Verification items for the finished model (mm, model axes). A direction names the side the tool comes from. Round coordinates to 2 decimals unless told otherwise and drop trailing zeros. Order: outer loops, then holes, each group sorted by start corner. A loop starts at its lowest first (then second) coordinate and runs counter-clockwise, first axis right, second up. Notation, with made-up numbers: M -20.75,-7.75 L 25.25,-7.75 A16 ccw 25.25,13.25 Z; hole C 50.25,8.5 d11. An arc over 180 degrees is marked long. Use one line per item in the form item = value. Start each with the question number.
Item 1: Tool access check on faces 1 (the flat face through (200, -12, -151)), 2 (the flat face through (0, -12, -152)). Record the directions out of +Z, -Z, +X, -X, +Y, -Y that give a thin tool (end or side, any length) a straight path to the whole face; none if there is none.
Item 2: Cross-section at C-C on z = -156. Enter the section's corners in (x, y), then the cut area to 4 significant figures.
Item 3: Thickness scan on probe 1 along X at (y, z) = (-23, -133.5); probe 2 along Z at (x, y) = (142.5, -8.25); probe 3 along Z at (x, y) = (99.5, -19.25). Record the ranges inside material, lowest first. Write a range as [from, to].
Item 4: Release check for a two-part mould opening along Z. For faces 3 (the flat face through (148, -12, -300)), 4 (the flat face through (99, -12, -151)), 5 (the flat face through (81, 0, -148)), 6 (the flat face through (149, -12, -100)) record: +Z half, -Z half, draft (parallel to the pull), parting line (faces both ways), or undercut.
Item 5: Cross-section at A-A on x = 161.5. Enter the section's corners in (y, z), then the cut area to 4 significant figures.
Item 6: Cross-section at B-B on y = -15.5. Enter the section's corners in (x, z).
from build123d import *

# Parameters (mm, degrees)
F0_W     = 300
F0_H     = 300
F0_W_2   = 101
F0_H_2   = 101
F1_DEPTH = 25
F2_SIZE  = 5


with BuildPart() as f1:
    # F0 (on Front) → F1 (new body)
    with BuildSketch(Plane.XZ):
        with Locations((150, -150)):
            Rectangle(F0_W, F0_H)
        with Locations((149.5, -150.5)):
            Rectangle(F0_W_2, F0_H_2, mode=Mode.SUBTRACT)
    extrude(amount=F1_DEPTH)

    # F2
    f2_edges = [f1.edges().sort_by_distance(p)[0] for p in [
        (0, -12.5, -300),
        (300, -12.5, -300),
        (300, -12.5, 0),
        (0, -12.5, 0),
        (200, -12.5, -201),
        (200, -12.5, -100),
        (99, -12.5, -100),
        (99, -12.5, -201),
    ]]
    chamfer(f2_edges, length=F2_SIZE)


solid = f1.part
Output values:
q1.face_1 = +Y, -Y
q1.face_2 = +Z, -Z, -X, +Y, -Y
q2.outline = M 0,-25 L 99,-25 L 99,0 L 0,0 Z; M 200,-25 L 300,-25 L 300,0 L 200,0 Z
q2.area = 4,975 mm2
q3.probe_1 = [0, 99], [200, 300]
q3.probe_2 = [-300, -201], [-100, 0]
q3.probe_3 = [-300, -196.5], [-104.5, 0]
q4.face_3 = -Z half
q4.face_4 = undercut
q4.face_5 = draft
q4.face_6 = undercut
q5.outline = M -25,-300 L 0,-300 L 0,-201 L -25,-201 Z; M -25,-100 L 0,-100 L 0,0 L -25,0 Z
q5.area = 4,975 mm2
q6.outline = M 0,-295 L 5,-300 L 295,-300 L 300,-295 L 300,-5 L 295,0 L 5,0 L 0,-5 Z; hole M 99,-196 L 104,-201 L 195,-201 L 200,-196 L 200,-105 L 195,-100 L 104,-100 L 99,-105 Z
